Source: CAD feature listing. Evaluate the final solid. Frame: model axes, mm. A direction names the side the tool comes from. Give positions to 0.01 mm unless a question says otherwise; leave off trailing zeros. Loops run counter-clockwise (first coordinate to the right, second up) from the corner with the lowest first, then second, coordinate; pieces in that order, holes last. Notation, with made-up numbers: M -32.75,-4 L -19.75,-4 A29 ccw -19.75,21 Z; hole C 60.5,-17 d7. An arc over 180 degrees is marked long. Put each result on its own line as item: value.
from build123d import *

# Parameters (mm, degrees)
SKETCH1_R           = 3
SKETCH1_R_2         = 2.5
BOSS_EXTRUDE1_DEPTH = 4
SKETCH2_R           = 1.3
CUT_EXTRUDE1_DEPTH  = 4
BOSS_EXTRUDE2_DEPTH = 4
SKETCH4_R           = 3
BOSS_EXTRUDE3_DEPTH = 4
SKETCH6_W           = 1.3795464
SKETCH6_H           = 7.5
CUT_EXTRUDE2_DEPTH  = 9
FILLET3_R           = 4
FILLET4_R           = 1


with BuildPart() as part:
    # Sketch1 → Boss-Extrude1 (new body)
    with BuildSketch(Plane(origin=(0, 0, 0), x_dir=(1, 0, 0), z_dir=(0, 1, 0))):
        with BuildLine():
            Line((-4.531642246, 17.7995776), (-7.838367177, 1.6))
            ThreePointArc((-7.838367177, 1.6), (0, -8), (7.838367177, 1.6))
            Line((7.838367177, 1.6), (4.531642246, 17.7995776))
            ThreePointArc((4.531642246, 17.7995776), (0, 21.499648), (-4.531642246, 17.7995776))
        make_face()
        with Locations(Location((0, 16.87456, 0), (0, 0, 270))):
            Circle(SKETCH1_R, mode=Mode.SUBTRACT)
        with Locations(Location((0, 0, 0), (0, 0, 270))):
            Circle(SKETCH1_R_2, mode=Mode.SUBTRACT)
    extrude(amount=BOSS_EXTRUDE1_DEPTH)

    # Sketch2 → Cut-Extrude1 (cut)
    with BuildSketch(Plane(origin=(0, 4, 0), x_dir=(1, 0, 0), z_dir=(0, 1, 0))):
        with Locations(Location((0, 6.35, 0), (0, 0, 270))):
            Circle(SKETCH2_R)
        with Locations(Location((6.35, 0, 0), (0, 0, 270))):
            Circle(SKETCH2_R)
        with Locations(Location((0, -6.35, 0), (0, 0, 270))):
            Circle(SKETCH2_R)
        with Locations(Location((-6.35, 0, 0), (0, 0, 270))):
            Circle(SKETCH2_R)
    extrude(amount=-CUT_EXTRUDE1_DEPTH, mode=Mode.SUBTRACT)

    # Sketch3 → Boss-Extrude2 (add)
    with BuildSketch(Plane(origin=(0, 4, 0), x_dir=(1, 0, 0), z_dir=(0, 1, 0))):
        with BuildLine():
            Line((-7.838367177, 1.6), (-6.8136721, 6.619960159))
            ThreePointArc((-6.8136721, 6.619960159), (0, -9.5), (6.8136721, 6.619960159))
            Line((6.8136721, 6.619960159), (7.838367177, 1.6))
            ThreePointArc((7.838367177, 1.6), (0, -8), (-7.838367177, 1.6))
        make_face()
    extrude(amount=-BOSS_EXTRUDE2_DEPTH)

    # Sketch4 → Boss-Extrude3 (add)
    with BuildSketch(Plane(origin=(0, 4, 0), x_dir=(1, 0, 0), z_dir=(0, 1, 0))):
        with BuildLine():
            Line((5, 35), (0, 35))
            Line((0, 35), (-5, 35))
            Line((-5, 35), (-5, 15.505102572))
            Line((-5, 15.505102572), (-4.531642246, 17.7995776))
            ThreePointArc((-4.531642246, 17.7995776), (0, 21.499648), (4.531642246, 17.7995776))
            Line((4.531642246, 17.7995776), (5, 15.505102572))
            Line((5, 15.505102572), (5, 35))
        make_face()
        with BuildLine():
            Line((5, 10), (5, 15.505102572))
            Line((5, 15.505102572), (4.531642246, 17.7995776))
            ThreePointArc((4.531642246, 17.7995776), (0, 21.499648), (-4.531642246, 17.7995776))
            Line((-4.531642246, 17.7995776), (-5, 15.505102572))
            Line((-5, 15.505102572), (-5, 10))
            Line((-5, 10), (0, 10))
            Line((0, 10), (5, 10))
        make_face()
        with Locations((0, 16.87456)):
            Circle(SKETCH4_R, mode=Mode.SUBTRACT)
        with Locations((0, 16.87456)):
            Circle(SKETCH4_R)
    extrude(amount=-BOSS_EXTRUDE3_DEPTH)

    # Sketch6 → Cut-Extrude2 (cut)
    with BuildSketch(Plane.XZ):
        with Locations((-4.3102268, -31.25)):
            Rectangle(SKETCH6_W, SKETCH6_H)
        Polygon((-3.6204536, -22.263472087), (-5, -15.505102572), (-5, -22.5), (-3.6204536, -22.5), align=None)
    extrude(amount=-CUT_EXTRUDE2_DEPTH, mode=Mode.SUBTRACT)

    # Fillet3
    fillet3_edges = [part.edges().sort_by_distance(p)[0] for p in [
        (5, 2, -35),
        (-3.6204536, 2, -35),
    ]]
    fillet(fillet3_edges, radius=FILLET3_R)

    # Fillet4
    fillet4_edges = [part.edges().sort_by_distance(p)[0] for p in [
        (-5, 2, -22.5),
        (-5, 2, -27.5),
    ]]
    fillet(fillet4_edges, radius=FILLET4_R)


solid = part.part
1. Draft query along Z for faces 6 (the cylindrical face through (7.64, 2.03, -0.17)), 7 (the cylindrical face through (-2.418, 2.028, -33.859)), 8 (the flat face through (0, 0, -8)). Return one class per face: pulls with the +Z half, pulls with the -Z half, needs draft (parallel to the pull), parting line crosses it, or undercut.
Found:
face 6: undercut
face 7: pulls with the -Z half
face 8: needs draft
2. Section query D-D (z = 6.35). Output: boundary loops of the cut face in (x, y), plus the area to 3 significant figures.
Found:
outline: M -7.07,0 L -1.3,0 L -1.3,4 L -7.07,4 Z; M 1.3,0 L 7.07,0 L 7.07,4 L 1.3,4 Z
area: 46.1 mm^2
3. Material intervals for line 1 (X direction, y = 1.7, z = 0); line 2 (Z direction, x = -0.75, y = 2.5); line 3 (Z direction, x = 0.5, y = 1.75), sorted ascending. Write a range as from..to.
Found:
line 1: -9.5..-7.65, -5.05..-2.5, 2.5..5.05, 7.65..9.5
line 2: -34.84..-7.41, -5.29..-2.38, 2.38..5.29, 7.41..9.47
line 3: -35..-7.55, -5.15..-2.45, 2.45..5.15, 7.55..9.49
4. Access query for faces 1 (the cylindrical face through (0.39, 2.03, -5.11)), 2 (the flat face through (0, 4, -8)), 3 (the flat face through (5, 2, -23)), 4 (the cylindrical face through (-4.715, 2.028, -22.801)), 5 (the flat face through (-3.62, 2, -29)). Directions: +Z, -Z, +X, -X, +Y, -Y. A direction counts if a zero-diameter tool reaches every point of the face in a straight line with its end or side. Return the directions, or none.
Found:
face 1: +Y, -Y
face 2: +Z, -Z, +X, -X, +Y
face 3: -Z, +X, +Y, -Y
face 4: -X, +Y, -Y
face 5: -Z, -X, +Y, -Y
5. Section query A-A (y = 2.75). Output: boundary loops of the cut face in (x, z).
Found:
outline: M -6.81,-6.62 L -3.62,-22.26 L -3.62,-22.5 L -4,-22.5 A1 ccw -5,-23.5 L -5,-26.5 A1 ccw -4,-27.5 L -3.62,-27.5 L -3.62,-31 A4 ccw 0.38,-35 L 1,-35 A4 ccw 5,-31 L 5,-15.51 L 6.81,-6.62 A9.5 ccw long Z; hole C -6.35,0 d2.6; hole C 0,0 d5; hole C 0,-6.35 d2.6; hole C 0,6.35 d2.6; hole C 6.35,0 d2.6
6. Section query B-B (z = 0). Output: boundary loops of the cut face in (x, y), plus the area to 3 significant figures.
Found:
outline: M -9.5,0 L -7.65,0 L -7.65,4 L -9.5,4 Z; M -5.05,0 L -2.5,0 L -2.5,4 L -5.05,4 Z; M 2.5,0 L 5.05,0 L 5.05,4 L 2.5,4 Z; M 7.65,0 L 9.5,0 L 9.5,4 L 7.65,4 Z
area: 35.2 mm^2
7. Contact query for flat-ended pins moving along their axis: P1, Ø1.5, axis at x = 6.5, y = 0.5, coming from the +Z side; P2, Ø1, axis at y = 1.5, z = -12.5, coming from the +X side; P3, Ø1.8, axis at y = 2.5, z = -29.5, coming from the -X side. Output: stop coordinate, or through.
Found:
P1: z = 7.56
P2: x = 5.72
P3: x = -3.62
8. Section query C-C (x = -6.35). Output: boundary loops of the cut face in (y, z).
Found:
outline: M 0,-8.89 L 4,-8.89 L 4,-1.3 L 0,-1.3 Z; M 0,1.3 L 4,1.3 L 4,7.07 L 0,7.07 Z
